Design review of the part built by this model. Coordinates are the model's own, in mm. A direction names the side the tool comes from. Coordinates: 2 decimals unless noted, no trailing zeros. Loops run counter-clockwise (first coordinate to the right, second up) from the corner with the lowest first, then second, coordinate; pieces in that order, holes last. Notation, with made-up numbers: (3, 74.5) - (59, 74.5) arc R19 ccw to (59, 107.5) - close; hole circle Ø3 at (82.25, -19.75). An arc over 180 degrees is marked (long way). Use one line per item in the form item = value. Start each with the question number.
(1) Add section C-C (y = -2.25). Count the separate pieces of the cut face and the enclosed holes in it, plus the area to 3 significant figures.
(2) Tool access review of faces 1 (the face through (150, -3, 175)), 2 (the face through (-3, -6.35, -163)): name each direction out of +Z, -Z, +X, -X, +Y, -Y from which nothing blocks a thin tool from reaching the whole face with its end or side.
(3) Add section B-B (z = 123). State the section outline as (x, y) points, plus the area to 3 significant figures.
(4) Add section A-A (x = 96). State the section outline as (y, z) points, plus the area to 3 significant figures.
(5) For L1, parallel to Z at x = 190, y = -2.75; L2, parallel to X at y = -3.5, z = 240; L3, parallel to Z at x = -110.5, y = -4, list the stretches that pass through material, from the lowest coordinate up.
(6) Clearance check with flat-ended pins moving along their axes: pin 1 Ø8 at (x, z) = (-79, -108) entering from +Y; pin 2 Ø3 at (y, z) = (-3.5, 238.5) entering from -X; pin 3 Ø1.9 at (y, z) = (-2, -234.5) entering from +X; pin 4 Ø3 at (x, y) = (-188.5, -3) entering from +Z. State where each tip first meets the part, or that it passes through.
(7) The part is to be moulded in two halves that separate along Z. For faces 3 (the face through (-150, -3, 175)), 4 (the face through (-3, 0, -163)), say which applies: pulls with the +Z half, pulls with the -Z half, needs draft (parallel to the pull), parting line crosses it, or undercut.
```python
from build123d import *

# Parameters (mm, degrees)
F0_R     = 2.01
F1_DEPTH = 6.35


with BuildPart() as f1:
    # F0 (on Front) → F1 (new body)
    with BuildSketch(Plane.XZ):
        Polygon((179.1715728753, -208), (190, -208), (200, -208), (200, 208), (190, 208), (179.1715728753, 208), (168.5857864376, 218.5857864376), (158, 229.1715728753), (158, 240), (158, 250), (-158, 250), (-158, 240), (-158, 229.1715728753), (-168.5857864376, 218.5857864376), (-179.1715728753, 208), (-190, 208), (-200, 208), (-200, -208), (-190, -208), (-179.1715728753, -208), (-168.5857864376, -218.5857864376), (-158, -229.1715728753), (-158, -240), (-158, -250), (158, -250), (158, -240), (158, -229.1715728753), (168.5857864376, -218.5857864376), align=None)
        with Locations((-190, -188)):
            Circle(F0_R, mode=Mode.SUBTRACT)
        with Locations((-138, -240)):
            Circle(F0_R, mode=Mode.SUBTRACT)
        with Locations((0, -240)):
            Circle(F0_R, mode=Mode.SUBTRACT)
        with Locations((138, -240)):
            Circle(F0_R, mode=Mode.SUBTRACT)
        with Locations((190, -188)):
            Circle(F0_R, mode=Mode.SUBTRACT)
        with Locations((-190, 0)):
            Circle(F0_R, mode=Mode.SUBTRACT)
        with Locations((-190, 188)):
            Circle(F0_R, mode=Mode.SUBTRACT)
        with Locations((-138, 240)):
            Circle(F0_R, mode=Mode.SUBTRACT)
        Polygon((-140, 185), (140, 185), (160, 165), (160, -115), (0, -115), (-160, -115), (-160, 165), align=None, mode=Mode.SUBTRACT)
        with Locations((190, 0)):
            Circle(F0_R, mode=Mode.SUBTRACT)
        with Locations((0, 240)):
            Circle(F0_R, mode=Mode.SUBTRACT)
        with Locations((138, 240)):
            Circle(F0_R, mode=Mode.SUBTRACT)
        with Locations((190, 188)):
            Circle(F0_R, mode=Mode.SUBTRACT)
    extrude(amount=F1_DEPTH)


solid = f1.part
```
Computed values:
q1.separate_pieces = 1
q1.enclosed_holes = 13
q1.area = 98,100 mm^2
q2.face_1 = +Y, -Y
q2.face_2 = +Z, -Z, +X, -X, -Y
q3.outline = (-200, -6.35) - (-160, -6.35) - (-160, 0) - (-200, 0) - close; (160, -6.35) - (200, -6.35) - (200, 0) - (160, 0) - close
q3.area = 508 mm^2
q4.outline = (-6.35, -250) - (0, -250) - (0, -115) - (-6.35, -115) - close; (-6.35, 185) - (0, 185) - (0, 250) - (-6.35, 250) - close
q4.area = 1,270 mm^2
q5.L1 = -208 to -190.01, -185.99 to -2.01, 2.01 to 185.99, 190.01 to 208
q5.L2 = -158 to -140.01, -135.99 to -2.01, 2.01 to 135.99, 140.01 to 158
q5.L3 = -250 to -115, 185 to 250
q6.pin_1 = through
q6.pin_2 = -158
q6.pin_3 = 158
q6.pin_4 = 208
q7.face_3 = undercut
q7.face_4 = needs draft
